from build123d import *

# Parameters (mm, degrees)
BOSS_EXTRUDE1_DEPTH                              = 2.6
SKETCH2_W                                        = 24.4
SKETCH2_H                                        = 408
BOSS_EXTRUDE2_DEPTH                              = 1.3
SKETCH3_W                                        = 2.8
SKETCH3_H                                        = 2.7
CUT_EXTRUDE1_DEPTH                               = 4.9
SKETCH4_W                                        = 1.3
SKETCH4_H                                        = 405.3
BOSS_EXTRUDE3_DEPTH                              = 5.3
SKETCH5_W                                        = 2.8
SKETCH5_H                                        = 2.7
CUT_EXTRUDE2_DEPTH                               = 7.6
SKETCH6_W                                        = 1.3
SKETCH6_H                                        = 405.3
BOSS_EXTRUDE4_DEPTH                              = 5.3
SKETCH7_W                                        = 18.8
SKETCH7_H                                        = 1.4
BOSS_EXTRUDE5_DEPTH                              = 8.6
SKETCH8_W                                        = 14
SKETCH8_H                                        = 6.5
CUT_EXTRUDE3_DEPTH                               = 10.9
CUT_EXTRUDE4_DEPTH                               = 2.3
CUT_EXTRUDE5_DEPTH                               = 2.3
CUT_EXTRUDE6_DEPTH                               = 2.3
CUT_EXTRUDE7_DEPTH                               = 2.3
CUT_EXTRUDE8_DEPTH                               = 10.9
CUT_EXTRUDE9_DEPTH                               = 2.6
DRAFT1_ANGLE                                     = 17.102728969
F_4_4_4_4_DIAMETER_HOLE1_D                       = 4.4
F_4_4_4_4_DIAMETER_HOLE1_DEPTH                   = 1.3
CBORE_FOR_M4_HEX_HEAD_MACHINE_SCREW1_D           = 4.4
CBORE_FOR_M4_HEX_HEAD_MACHINE_SCREW1_DEPTH       = 3.9
CBORE_FOR_M4_HEX_HEAD_MACHINE_SCREW1_CBORE_D     = 7.5
CBORE_FOR_M4_HEX_HEAD_MACHINE_SCREW1_CBORE_DEPTH = 1
SCALE1_SCALE                                     = 0.25


with BuildPart() as part:
    # Sketch1 → Boss-Extrude1 (new body)
    with BuildSketch(Plane.XZ.offset(0.6)):
        with BuildLine():
            Line((3.75, 390.2), (3.140289704, 397.947144852))
            ThreePointArc((3.140289704, 397.947144852), (0, 400.85), (-3.140289704, 397.947144852))
            Line((-3.140289704, 397.947144852), (-3.75, 390.2))
            ThreePointArc((-3.75, 390.2), (0, 386.45), (3.75, 390.2))
        make_face()
    extrude(amount=-BOSS_EXTRUDE1_DEPTH)

    # Sketch2 → Boss-Extrude2 (add)
    with BuildSketch(Plane.XZ.offset(-2)):
        with Locations((0, 204)):
            Rectangle(SKETCH2_W, SKETCH2_H)
        with BuildLine():
            Line((-2.05, 392.9), (2.05, 392.9))
            ThreePointArc((2.05, 392.9), (4.75, 390.2), (2.05, 387.5))
            Line((2.05, 387.5), (-2.05, 387.5))
            ThreePointArc((-2.05, 387.5), (-4.75, 390.2), (-2.05, 392.9))
        make_face(mode=Mode.SUBTRACT)
    extrude(amount=-BOSS_EXTRUDE2_DEPTH)

    # Sketch3 → Cut-Extrude1 (cut, through all)
    with BuildSketch(Plane(origin=(0, 3.3, 0), x_dir=(-1, 0, 0), z_dir=(0, 1, 0))):
        with Locations((-10.8, 406.65)):
            Rectangle(SKETCH3_W, SKETCH3_H)
    extrude(amount=-CUT_EXTRUDE1_DEPTH, mode=Mode.SUBTRACT)

    # Sketch4 → Boss-Extrude3 (add)
    with BuildSketch(Plane.XZ.offset(-2)):
        with Locations((11.55, 202.65)):
            Rectangle(SKETCH4_W, SKETCH4_H)
    extrude(amount=BOSS_EXTRUDE3_DEPTH)

    # Sketch5 → Cut-Extrude2 (cut, through all)
    with BuildSketch(Plane(origin=(0, 3.3, 0), x_dir=(-1, 0, 0), z_dir=(0, 1, 0))):
        with Locations((10.8, 406.65)):
            Rectangle(SKETCH5_W, SKETCH5_H)
    extrude(amount=-CUT_EXTRUDE2_DEPTH, mode=Mode.SUBTRACT)

    # Sketch6 → Boss-Extrude4 (add)
    with BuildSketch(Plane.XZ.offset(-2)):
        with Locations((-11.55, 202.65)):
            Rectangle(SKETCH6_W, SKETCH6_H)
    extrude(amount=BOSS_EXTRUDE4_DEPTH)

    # Sketch7 → Boss-Extrude5 (add)
    with BuildSketch(Plane.XZ.offset(-2)):
        with Locations((0, 407.3)):
            Rectangle(SKETCH7_W, SKETCH7_H)
    extrude(amount=BOSS_EXTRUDE5_DEPTH)

    # Sketch8 → Cut-Extrude3 (cut, through all)
    with BuildSketch(Plane(origin=(0, 3.3, 0), x_dir=(-1, 0, 0), z_dir=(0, 1, 0))):
        with Locations((0, 3.25)):
            Rectangle(SKETCH8_W, SKETCH8_H)
    extrude(amount=-CUT_EXTRUDE3_DEPTH, mode=Mode.SUBTRACT)

    # Sketch9 → Cut-Extrude4 (cut, through all)
    with BuildSketch(Plane.XZ.offset(-2)):
        with BuildLine():
            Line((2.55, 375.200000014), (-2.55, 375.200000014))
            ThreePointArc((-2.55, 375.200000014), (-4.75, 373.000000014), (-2.55, 370.800000014))
            Line((-2.55, 370.800000014), (2.55, 370.800000014))
            ThreePointArc((2.55, 370.800000014), (4.75, 373.000000014), (2.55, 375.200000014))
        make_face()
    extrude(amount=-CUT_EXTRUDE4_DEPTH, mode=Mode.SUBTRACT)

    # Sketch10 → Cut-Extrude5 (cut, through all)
    with BuildSketch(Plane.XZ.offset(-2)):
        with BuildLine():
            Line((-2.549860329, 242.799983225), (2.550139671, 242.8))
            ThreePointArc((2.550139671, 242.8), (4.750132435, 245.000007236), (2.550125198, 247.2))
            Line((2.550125198, 247.2), (-2.549874802, 247.199983225))
            ThreePointArc((-2.549874802, 247.199983225), (-4.749867565, 244.999975989), (-2.549860329, 242.799983225))
        make_face()
    extrude(amount=-CUT_EXTRUDE5_DEPTH, mode=Mode.SUBTRACT)

    # Sketch11 → Cut-Extrude6 (cut, through all)
    with BuildSketch(Plane.XZ.offset(-2)):
        with BuildLine():
            Line((2.200125198, 309.95), (2.200125198, 315.05))
            ThreePointArc((2.200125198, 315.05), (0.000125198, 317.25), (-2.199874802, 315.05))
            Line((-2.199874802, 315.05), (-2.199874802, 309.95))
            ThreePointArc((-2.199874802, 309.95), (0.000125198, 307.75), (2.200125198, 309.95))
        make_face()
    extrude(amount=-CUT_EXTRUDE6_DEPTH, mode=Mode.SUBTRACT)

    # Sketch12 → Cut-Extrude7 (cut, through all)
    with BuildSketch(Plane.XZ.offset(-2)):
        with BuildLine():
            Line((2.200125198, 28.45), (2.200125198, 33.55))
            ThreePointArc((2.200125198, 33.55), (0.000125198, 35.75), (-2.199874802, 33.55))
            Line((-2.199874802, 33.55), (-2.199874802, 28.45))
            ThreePointArc((-2.199874802, 28.45), (0.000125198, 26.25), (2.200125198, 28.45))
        make_face()
    extrude(amount=-CUT_EXTRUDE7_DEPTH, mode=Mode.SUBTRACT)

    # Sketch13 → Cut-Extrude8 (cut, through all)
    with BuildSketch(Plane(origin=(0, 3.3, 0), x_dir=(-1, 0, 0), z_dir=(0, 1, 0))):
        with BuildLine():
            Line((2.549874802, 55.2), (-2.550125198, 55.2))
            ThreePointArc((-2.550125198, 55.2), (-4.750125198, 53), (-2.550125198, 50.8))
            Line((-2.550125198, 50.8), (2.549874802, 50.8))
            ThreePointArc((2.549874802, 50.8), (4.749874802, 53), (2.549874802, 55.2))
        make_face()
    extrude(amount=-CUT_EXTRUDE8_DEPTH, mode=Mode.SUBTRACT)

    # Sketch14 → Cut-Extrude9 (cut)
    with BuildSketch(Plane.XZ.offset(0.6)):
        Polygon((0.6, 397.1), (2.2, 397.1), (2.2, 398.3), (0.6, 398.3), (0.6, 399.9), (-0.6, 399.9), (-0.6, 398.3), (-2.2, 398.3), (-2.2, 397.1), (-0.6, 397.1), (-0.6, 395.5), (0.6, 395.5), align=None)
    extrude(amount=-CUT_EXTRUDE9_DEPTH, mode=Mode.SUBTRACT)

    # Draft1
    draft1_faces = [part.faces().sort_by_distance(p)[0] for p in [
        (-7, 2.65, 3.25),
        (7, 2.65, 3.25),
    ]]
    draft(draft1_faces, Plane(origin=(-7, -6.6, 6.5), x_dir=(0, -1, 0), z_dir=(0, 0, -1)), DRAFT1_ANGLE)

    # Ø4.4 (4.4) Diameter Hole1
    with Locations(Plane(origin=(0, 2, 0), x_dir=(-1, 0, 0), z_dir=(0, -1, 0))):
        with Locations((-0.000125198, -62), (-0.000125198, -254), (0, -382)):
            Hole(F_4_4_4_4_DIAMETER_HOLE1_D / 2, depth=F_4_4_4_4_DIAMETER_HOLE1_DEPTH)

    # CBORE for M4 Hex Head Machine Screw1
    with Locations(Plane(origin=(0, -0.6, 0), x_dir=(-1, 0, 0), z_dir=(0, -1, 0))):
        with Locations((0, -390.2)):
            CounterBoreHole(CBORE_FOR_M4_HEX_HEAD_MACHINE_SCREW1_D / 2, CBORE_FOR_M4_HEX_HEAD_MACHINE_SCREW1_CBORE_D / 2, CBORE_FOR_M4_HEX_HEAD_MACHINE_SCREW1_CBORE_DEPTH, depth=CBORE_FOR_M4_HEX_HEAD_MACHINE_SCREW1_DEPTH)


with BuildPart() as part_1:
    # Scale1: scaled about (-1.622e-06, 1.572421019, 208.139009322)
    add(part.part.scale(SCALE1_SCALE).moved(Location((-1.217e-06, 1.179315764, 156.104256991))))


solid = part_1.part
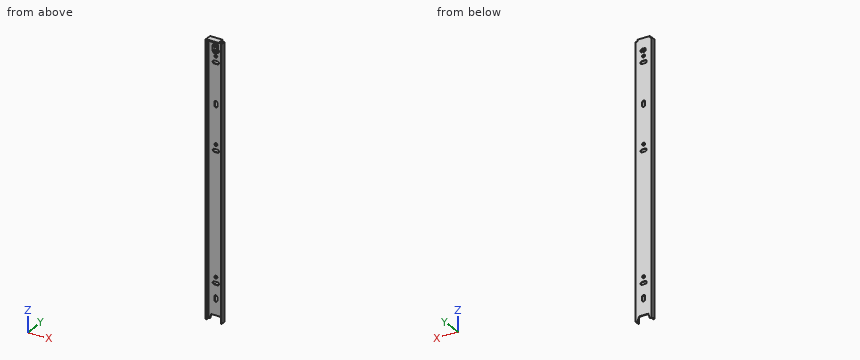
The listing builds one solid part. Answer for the finished solid, in the listing's coordinates (mm). Round coordinates to 2 decimals unless told otherwise and drop trailing zeros. Write each loop counter-clockwise with the first axis right and the second up, starting at its lowest first coordinate (ties: lowest second). Pieces come first, ordered by that corner, then holes. Notation, with made-up numbers: (-5.75, -33.5) - (18.25, -33.5) arc R5 ccw to (18.25, -29.5) - close; hole circle Ø3 at (-24, 59). An arc over 180 degrees is marked (long way). Use a Markdown table: item, result. Add a question column.
1. Flat-ended cylindrical pins translate along their axes: P1, Ø0.5, axis at y = 0.5, z = 258, coming from the -X side; P2, Ø1.2, axis at x = 0, z = 255.5, coming from the -Y side. Find the tip coordinate at first contact, or state that the pin passes through.
2. The part is cut by section A-A (z = 178). Write down the section's boundary in (x, y) (3 decimals).
3. Consider line 1 (X direction, y = 1.15, z = 170) (3 decimals); line 2 (Z direction, x = 1, y = 1.95); line 3 (Z direction, x = 1, y = 0.5). Determine where each line is inside the solid, lowest interval first.
Reported:
| question | item | result |
|---|---|---|
| 1 | P1 | x = -2.35 |
| 1 | P2 | y = 1.03 |
| 2 | outline | (-3.05, 0.354) - (-2.725, 0.354) - (-2.725, 1.679) - (2.725, 1.679) - (2.725, 0.354) - (3.05, 0.354) - (3.05, 2.004) - (-3.05, 2.004) - close |
| 3 | line 1 | -3.05 to -2.725, 2.725 to 3.05 |
| 3 | line 2 | 157.73 to 168.94, 169.77 to 216.94, 217.77 to 248.94, 249.77 to 253.19, 254.12 to 258.1 |
| 3 | line 3 | 257.75 to 258.1 |
